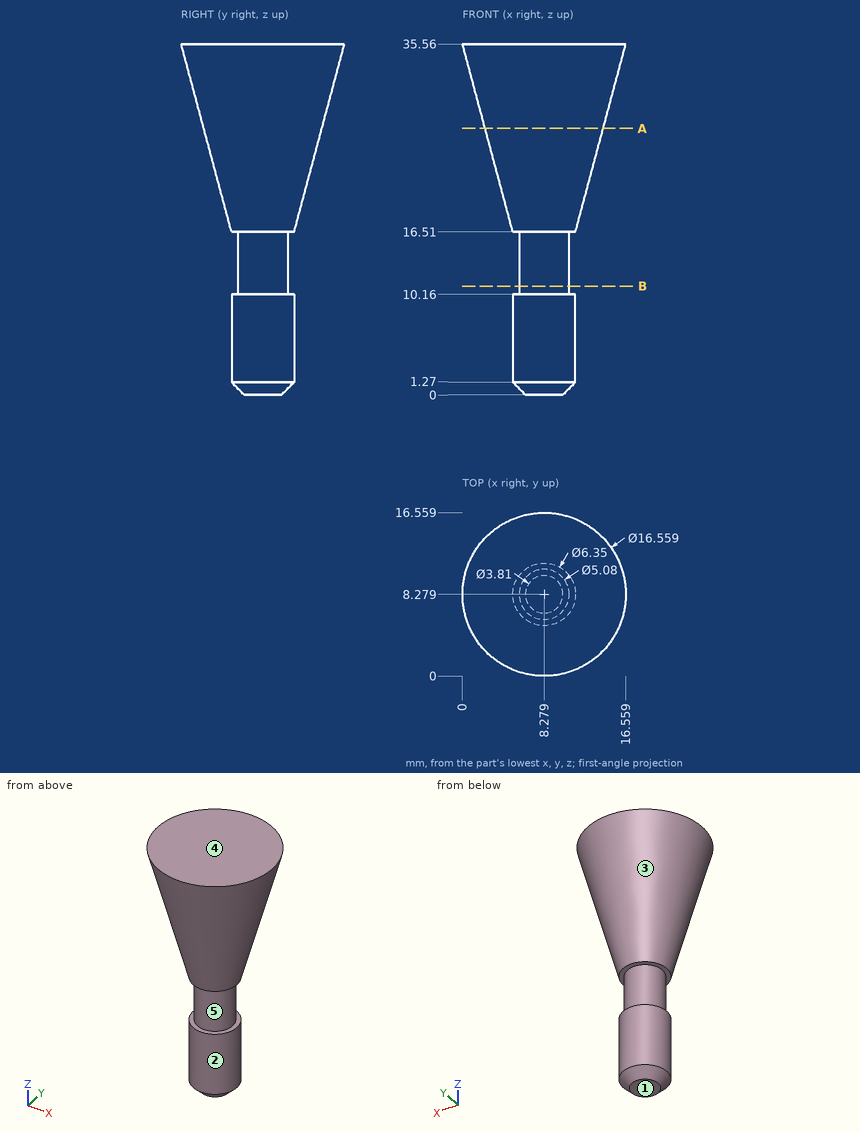
Input: dimensioned drawing with shaded views. Units: mm. Origin: part minimum x, y, z. A direction names the side the tool comes from. Coordinates: 2 decimals unless noted, no trailing zeros. Order: outer loops, then holes, each group sorted by start corner. A loop starts at its lowest first (then second) coordinate and runs counter-clockwise, first axis right, second up.
1. Contact query for flat-ended pins moving along their axis: P1, Ø1.5, axis at y = 5.5, z = 31, coming from the +X side; P2, Ø1, axis at x = 6, z = 10, coming from the -Y side; P3, Ø1, axis at x = 3, z = 28.5, coming from the -Y side (1 decimal). Output: stop coordinate, or through.
Checked values:
P1: stops at x = 15.12
P2: stops at y = 5.65
P3: stops at y = 4
2. Ray query, line 1 along Z through (x, y) = (11, 8.25) (1 decimal); line 2 along X through (y, z) = (10, 11.5); line 3 along Y through (x, z) = (4.75, 30.5) (1 decimal). Return the intervals inside material, ascending.
Checked values:
line 1: z = 0.8 to 10.2, 16.5 to 35.6
line 2: x = 6.41 to 10.15
line 3: y = 2.3 to 14.2
3. Cut plane A-A, the plane z = 27. Return loops of the section in (x, y) (1 decimal), plus the area to 3 significant figures.
Checked values:
outline: circle Ø12 at (8.3, 8.3)
area: 113 mm2
4. Access query for the marked faces 1 and 2. Directions: +Z, -Z, +X, -X, +Y, -Y. A direction counts if a zero-diameter tool reaches every point of the face in a straight line with its end or side. Return the directions, or none.
Checked values:
face 1: -Z, +X, -X, +Y, -Y
face 2: -Z
5. Cut plane B-B, the plane z = 11. Return loops of the section in (x, y), plus the area to 3 significant figures.
Checked values:
outline: circle Ø5.08 at (8.28, 8.28)
area: 20.3 mm2
6. Draft query along Z for the marked faces 3, 4 and 5. Return one class per face: +Z half, -Z half, draft (parallel to the pull), parting line (faces both ways), or undercut.
Checked values:
face 3: -Z half
face 4: +Z half
face 5: undercut
